```python
from build123d import *

# Parameters (mm, degrees)
SKETCH1_R           = 41.402
SKETCH1_R_2         = 36.6395
BOSS_EXTRUDE1_DEPTH = 25.4
CHAMFER1_SIZE       = 1.5875
SKETCH2_W           = 12.7
SKETCH2_H           = 4.7625
CUT_EXTRUDE1_DEPTH  = 64.823281081
CIRPATTERN1_COUNT   = 15


with BuildPart() as part:
    # Sketch1 → Boss-Extrude1 (new body)
    with BuildSketch(Plane.XY):
        Circle(SKETCH1_R)
        Circle(SKETCH1_R_2, mode=Mode.SUBTRACT)
    extrude(amount=-BOSS_EXTRUDE1_DEPTH)

    # Chamfer1
    chamfer1_edges = [part.edges().sort_by_distance(p)[0] for p in [
        (-41.402, 0, 0),
        (-41.402, 0, -25.4),
        (-36.6395, 0, -25.4),
        (-36.6395, 0, 0),
    ]]
    chamfer(chamfer1_edges, length=CHAMFER1_SIZE)

    # Sketch2 → Cut-Extrude1 (cut, through all)
    with BuildSketch(Plane(origin=(0, 0, 0), x_dir=(0, 0, -1), z_dir=(1, 0, 0))):
        Rectangle(SKETCH2_W, SKETCH2_H)
    cut_extrude1 = extrude(amount=-CUT_EXTRUDE1_DEPTH, mode=Mode.SUBTRACT)

    # CirPattern1: Cut-Extrude1 ×15 about axis
    cirpattern1_axis = Axis((0, 0, 0), (0, 0, 1))
    for i in range(1, CIRPATTERN1_COUNT):
        add(cut_extrude1.rotate(cirpattern1_axis, i * 360 / CIRPATTERN1_COUNT), mode=Mode.SUBTRACT)


solid = part.part
```
For this review, take the finished solid that the model builds, in its own axes (mm). A direction names the side the tool comes from. Give positions to 0.01 mm unless a question says otherwise; leave off trailing zeros. Order: outer loops, then holes, each group sorted by start corner. A loop starts at its lowest first (then second) coordinate and runs counter-clockwise, first axis right, second up.
1) The part is to be moulded in two halves that separate along Y. For faces 6 (the face through (11.64, 35.59, -0.78)), 7 (the face through (6.436, -38.452, -3.131)), 8 (the face through (-20.22, 35.2, -0.78)), say which applies: released by +Y, released by -Y, zero draft, split by the parting line, or undercut.
2) For faces 1 (the face through (37.57, 10.42, -3.13)), 2 (the face through (11.5, -35.64, -0.78)), 3 (the face through (21.52, -32.51, -3.13)), 4 (the face through (-39, -2.381, -3)), 5 (the face through (-14.3, 36.3, -3.1)), list the 3-axis set-ups (+Z, -Z, +X, -X, +Y, -Y) from which the entire face can be reached by the end or side of a thin tool; tool diameter is ignored.
3) Wall thickness on line 1 (Y direction, x = 0, z = -16.75); line 2 (Y direction, x = 21.5, z = -17); line 3 (X direction, y = -10, z = -23.75): over which ranges is each line inside the solid? List them lowest first.
4) Take a section at D-D (z = -4.5). State how many separate pieces and enclosed holes the cut face has, then the cut area to 3 significant figures.
5) Take a section at A-A (x = 0). Give the boundary of the cut face in (y, z).
6) Take a section at B-B (y = 0). Give the boundary of the cut face in (x, z), then the cut area to 3 significant figures.
7) Insertion check: pin 1 (4 mm diameter, centred on x = 4.5, y = 38, fed in from +Z); pin 2 (3 mm diameter, centred on x = 39, y = 9, fed in from +Z); pin 3 (1 mm diameter, centred on y = -31, z = -22, fed in from +X); pin 4 (3 mm diameter, centred on x = -2, z = -17, fed in from +Y). Each pin has a flat end and moves straight along its axis. Give the tip position at first contact, or say it passes through.
8) Take a section at C-C (z = -13.25). Give the boundary of the cut face in (x, y).
Derived:
1. face 6: undercut
1. face 7: released by -Y
1. face 8: released by +Y
2. face 1: +Z, +X
2. face 2: +Z
2. face 3: +Z, -Y
2. face 4: +Z, -X
2. face 5: +Z, +Y
3. line 1: y = -41.4 to -36.64, 36.64 to 41.4
3. line 2: y = -35.38 to -29.67, 29.67 to 35.38
3. line 3: x = -40.18 to -35.25, 35.25 to 40.18
4. separate pieces: 15
4. enclosed holes: 0
4. area: 827 mm2
5. outline: (-41.4, -23.81) - (-39.81, -25.4) - (-38.23, -25.4) - (-36.64, -23.81) - (-36.64, -1.59) - (-38.23, 0) - (-39.81, 0) - (-41.4, -1.59) - close; (36.64, -23.81) - (38.23, -25.4) - (39.81, -25.4) - (41.4, -23.81) - (41.4, -1.59) - (39.81, 0) - (38.23, 0) - (36.64, -1.59) - close
6. outline: (-41.4, -23.81) - (-39.81, -25.4) - (-38.23, -25.4) - (-36.64, -23.81) - (-36.64, -6.35) - (-41.4, -6.35) - close; (36.64, -23.81) - (38.23, -25.4) - (39.81, -25.4) - (41.4, -23.81) - (41.4, -1.59) - (39.81, 0) - (38.23, 0) - (36.64, -1.59) - close
6. area: 204 mm2
7. pin 1: stops at z = 0
7. pin 2: stops at z = -6.35
7. pin 3: stops at x = 28
7. pin 4: stops at y = 41.4
8. outline: circle Ø82.8 at (0, 0); hole circle Ø73.28 at (0, 0)
